from build123d import *

# Parameters (mm, degrees)
EXTRUDE_THIN1_DEPTH = 450
SKETCH2_R           = 5
CUT_EXTRUDE1_DEPTH  = 893
FILLET1_R           = 10


with BuildPart() as part:
    # Sketch1 → Extrude-Thin1 (new body, symmetric)
    with BuildSketch(Plane.XY):
        Polygon((-250, 50), (-250, 0), (630, 0), (630, 50), (636, 50), (636, -6), (-256, -6), (-256, 50), align=None)
    extrude(amount=EXTRUDE_THIN1_DEPTH, both=True)

    # Sketch2 → Cut-Extrude1 (cut, through all)
    with BuildSketch(Plane(origin=(636, 0, 0), x_dir=(0, 0, -1), z_dir=(1, 0, 0))):
        with Locations((420, 24)):
            Circle(SKETCH2_R)
        with BuildLine():
            Line((20, 19), (-180, 19))
            ThreePointArc((-180, 19), (-185, 24), (-180, 29))
            Line((-180, 29), (20, 29))
            ThreePointArc((20, 29), (25, 24), (20, 19))
        make_face()
    extrude(amount=-CUT_EXTRUDE1_DEPTH, mode=Mode.SUBTRACT)

    # Fillet1
    fillet1_edges = [part.edges().sort_by_distance(p)[0] for p in [
        (-253, 50, 450),
        (-253, 50, -450),
        (633, 50, 450),
        (633, 50, -450),
    ]]
    fillet(fillet1_edges, radius=FILLET1_R)


solid = part.part
Read the model definition and answer for the solid it produces. Units are mm, in the model's axes. A direction names the side the tool comes from. Coordinates: 2 decimals unless noted, no trailing zeros. Write each loop counter-clockwise with the first axis right and the second up, starting at its lowest first coordinate (ties: lowest second). Pieces come first, ordered by that corner, then holes. Notation, with made-up numbers: (26, 21) -> (58, 21) arc R17 ccw to (58, 43) -> close; hole circle Ø9 at (-14, 76.5). An arc over 180 degrees is marked (long way). Return JSON: item names as keys, results as strings.
(1) Which of the six approach directions +Z, -Z, +X, -X, +Y, -Y give full straight-line access (tool end or side, diameter ignored) to faces 4 (the flat face through (636, 16, 6)), 5 (the flat face through (-250, 31, 6))?
Answers below:
{"face 4": "+Z, -Z, +X, +Y, -Y", "face 5": "+Z, -Z, +Y"}
(2) The part is cut by section C-C on x = 159. Give the vertices of the cut face in (y, z).
Answers below:
{"outline": "(-6, -450) -> (0, -450) -> (0, 450) -> (-6, 450) -> close"}
(3) Each of these flat-tipped pins is pushed along its axis until it touches: P1, Ø8, axis at x = 308, z = -156, coming from the +Y side; P2, Ø9, axis at y = 24, z = -420, coming from the -X side. Where does it stop, or does it pass through?
Answers below:
{"P1": "y = 0", "P2": "through"}
(4) The part is cut by section B-B on z = -97. Give the vertices of the cut face in (x, y).
Answers below:
{"outline": "(-256, -6) -> (636, -6) -> (636, 50) -> (630, 50) -> (630, 0) -> (-250, 0) -> (-250, 50) -> (-256, 50) -> close"}
(5) For a pull along X with two mould halves and no side action, classify faces 1 (the flat face through (192, -3, -450)), 2 (the flat face through (-256, 15, 6)), 3 (the flat face through (184, 0, 6)) as pulls with the +X half, pulls with the -X half, needs draft (parallel to the pull), parting line crosses it, or undercut.
Answers below:
{"face 1": "needs draft", "face 2": "pulls with the -X half", "face 3": "undercut"}
(6) Consider line 1 along X through (y, z) = (6, -365); line 2 along Y through (x, z) = (-254.3, -420); line 3 along Y through (x, z) = (-90, -50). Determine where each line is inside the solid, lowest interval first. Write a range as from..to.
Answers below:
{"line 1": "-256..-250, 630..636", "line 2": "-6..19, 29..50", "line 3": "-6..0"}
(7) The part is cut by section A-A on z = 30.5. Give the vertices of the cut face in (x, y), then the cut area to 3 significant figures.
Answers below:
{"outline": "(-256, -6) -> (636, -6) -> (636, 19) -> (630, 19) -> (630, 0) -> (-250, 0) -> (-250, 19) -> (-256, 19) -> close; (-256, 29) -> (-250, 29) -> (-250, 50) -> (-256, 50) -> close; (630, 29) -> (636, 29) -> (636, 50) -> (630, 50) -> close", "area": "5,830 mm^2"}
